Source: three-view drawing plus pictorial views. Frame: mm from the lowest corner of the part. A direction names the side the tool comes from. Give positions to 0.01 mm unless a question says otherwise; leave off trailing zeros. Loops run counter-clockwise (first coordinate to the right, second up) from the corner with the lowest first, then second, coordinate; pieces in that order, holes last. Notation, with made-up numbers: M -7,0.25 L 19,0.25 A19 ccw 19,25.25 Z; hole C 89,79.5 d9. An arc over 180 degrees is marked long. Answer as a JSON object with one key per item and string values. Group by question number.
1) Ray query, L1, parallel to Z at x = 13.15, y = 0.5; L2, parallel to Z at x = 21.25, y = 23.5; L3, parallel to Y at x = 13, z = 14.25. Return the intervals inside material, ascending.
2) First-contact query: P1, Ø1.2, axis at x = 13.15, z = 4, coming from the -Y side; P2, Ø5, axis at y = 20, z = 10.5, coming from the -X side; P3, Ø2, axis at x = 10.5, y = 21.5, coming from the -Z side; P4, Ø6, axis at x = 20, z = 13, coming from the +Y side. Flat tips, straight axial feed; report the tip coordinate or a pass-through.
3) Access query for the marked faces 1 and 2. Directions: +Z, -Z, +X, -X, +Y, -Y. A direction counts if a zero-diameter tool reaches every point of the face in a straight line with its end or side. Return the directions, or none.
4) Section query A-A on z = 4. Return loops of the section in (x, y), plus the area to 3 significant figures.
5) Section query D-D on y = 7. Return loops of the section in (x, z).
6) Section query B-B on x = 13.15. Return loops of the section in (y, z).
7) Section query C-C on y = 15.15. Return loops of the section in (x, z).
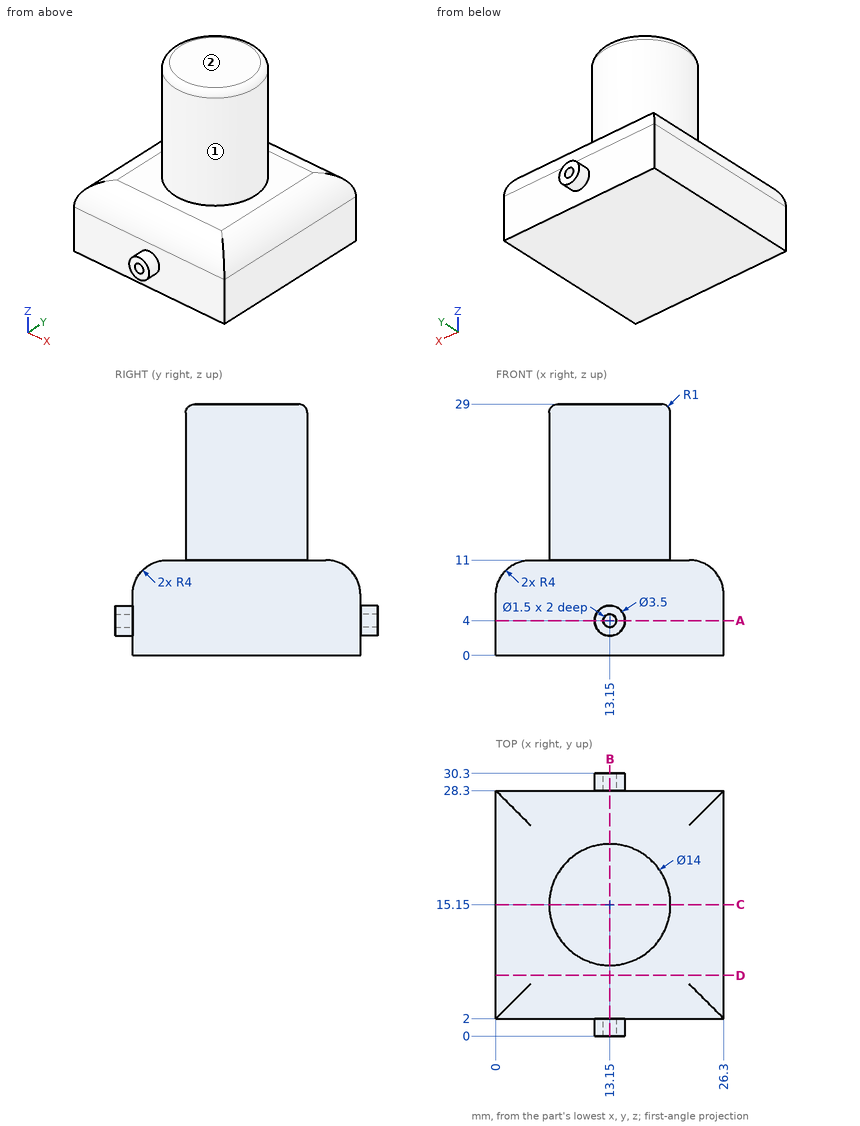
Output:
{
 "1": {"L1": "z = 2.25 to 3.25, 4.75 to 5.75", "L2": "z = 0 to 11", "L3": "y = 8.15 to 22.15"},
 "2": {"P1": "stops at y = 2", "P2": "stops at x = 0.13", "P3": "stops at z = 0", "P4": "stops at y = 26.95"},
 "3": {"face 1": "+Z", "face 2": "+Z, +X, -X, +Y, -Y"},
 "4": {"outline": "M 0,2 L 11.4,2 L 11.4,0 L 12.4,0 L 12.4,2 L 13.9,2 L 13.9,0 L 14.9,0 L 14.9,2 L 26.3,2 L 26.3,28.3 L 14.9,28.3 L 14.9,30.3 L 13.9,30.3 L 13.9,28.3 L 12.4,28.3 L 12.4,30.3 L 11.4,30.3 L 11.4,28.3 L 0,28.3 Z", "area": "700 mm^2"},
 "5": {"outline": "M 0,0 L 26.3,0 L 26.3,7 A4 ccw 22.3,11 L 4,11 A4 ccw 0,7 Z"},
 "6": {"outline": "M 0,2.25 L 2,2.25 L 2,0 L 28.3,0 L 28.3,2.25 L 30.3,2.25 L 30.3,3.25 L 28.3,3.25 L 28.3,4.75 L 30.3,4.75 L 30.3,5.75 L 28.3,5.75 L 28.3,7 A4 ccw 24.3,11 L 22.15,11 L 22.15,28 A1 ccw 21.15,29 L 9.15,29 A1 ccw 8.15,28 L 8.15,11 L 6,11 A4 ccw 2,7 L 2,5.75 L 0,5.75 L 0,4.75 L 2,4.75 L 2,3.25 L 0,3.25 Z"},
 "7": {"outline": "M 0,0 L 26.3,0 L 26.3,7 A4 ccw 22.3,11 L 20.15,11 L 20.15,28 A1 ccw 19.15,29 L 7.15,29 A1 ccw 6.15,28 L 6.15,11 L 4,11 A4 ccw 0,7 Z"}
}
